from build123d import *
from OCP.BRepFilletAPI import BRepFilletAPI_MakeChamfer

# Parameters (mm, degrees)
BOSS_EXTRUDE1_DEPTH           = 6
FILLET1_R                     = 3
LPATTERN1_COUNT               = 2
LPATTERN1_PITCH               = 19
CSK_FOR_M4_SFHCS1_D           = 4.5
CSK_FOR_M4_SFHCS1_CSINK_D     = 8.96
CSK_FOR_M4_SFHCS1_CSINK_ANGLE = 90
FILLET2_R                     = 8
FILLET3_R                     = 2
CHAMFER1_SIZE                 = 3
CHAMFER1_SIZE2                = 1.732050808


# Some blends are built 0.0001 mm under size
with BuildPart() as part:
    # Sketch1 → Boss-Extrude1 (new body)
    with BuildSketch(Plane(origin=(0, 0, 0), x_dir=(1, 0, 0), z_dir=(0, 1, 0))):
        Polygon((10, 20), (16.5, 20), (16.5, 17), (10, 17), (10, 2), (16.5, 2), (16.5, -2), (10, -2), (10, -17), (16.5, -17), (16.5, -20), (10, -20), (-10, -20), (-10, 20), align=None)
    extrude(amount=BOSS_EXTRUDE1_DEPTH)

    # Fillet1
    fillet1_edges = [part.edges().sort_by_distance(p)[0] for p in [
        (16.5, 6, -18.5),
        (16.5, 0, -18.5),
        (16.5, 0, 0),
        (16.5, 0, 18.5),
        (16.5, 6, 0),
        (16.5, 6, 18.5),
    ]]
    fillet(fillet1_edges, radius=FILLET1_R - 0.0001)  # a hair under: the kernel refuses the full size

    # Sketch2 → Revolve1 (revolve)
    with BuildSketch(Plane(origin=(13.5, 0, 0), x_dir=(0, 0, -1), z_dir=(1, 0, 0))):
        with BuildLine():
            Line((-2, 3), (-2, 5.5))
            ThreePointArc((-2, 5.5), (-3.767766953, 4.767766953), (-4.5, 3))
            Line((-4.5, 3), (-2, 3))
        make_face()
    revolve1 = revolve(axis=Axis((13.5, 3, 2), (0, 0, 1)))

    # LPattern1: Revolve1 ×2
    with Locations(*[(0, 0, -i * LPATTERN1_PITCH) for i in range(1, LPATTERN1_COUNT)]):
        add(revolve1)

    # Mirror1: Revolve1 across plane
    add(revolve1.mirror(Plane.XY))

    # Mirror1 copy 1 sketch → Mirror1 copy 1 (revolve)
    with BuildSketch(Plane(origin=(13.5, 0, 19), x_dir=(0, 0, 1), z_dir=(1, 0, 0))):
        with BuildLine():
            Line((-2, -3), (-2, -5.5))
            ThreePointArc((-2, -5.5), (-3.767766953, -4.767766953), (-4.5, -3))
            Line((-4.5, -3), (-2, -3))
        make_face()
    revolve(axis=Axis((13.5, 3, 17), (0, 0, 1)))

    # CSK for M4 SFHCS1 (through all)
    with Locations(Plane(origin=(-2.75, 6, -10), x_dir=(0, 0, 1), z_dir=(0, 1, 0))):
        with Locations((0, 0), (20, 0)):
            CounterSinkHole(CSK_FOR_M4_SFHCS1_D / 2, CSK_FOR_M4_SFHCS1_CSINK_D / 2, counter_sink_angle=CSK_FOR_M4_SFHCS1_CSINK_ANGLE)

    # Fillet2
    fillet2_edges = [part.edges().sort_by_distance(p)[0] for p in [
        (-10, 3, -20),
        (-10, 3, 20),
    ]]
    fillet(fillet2_edges, radius=FILLET2_R)

    # Fillet3
    # the kernel refuses this fillet: 2 mm, written as the material it takes off along each edge
    with BuildSketch(Plane(origin=(18.5001, 6, 20), x_dir=(0, 0, -1), z_dir=(-1, 0, 0))) as fillet3_piece_1:
        with BuildLine():
            CenterArc((FILLET3_R, FILLET3_R), FILLET3_R, 180, 90)
            Line((0, FILLET3_R), (0, 0))
            Line((0, 0), (FILLET3_R, 0))
        make_face()
    extrude(amount=20.5001, mode=Mode.SUBTRACT)
    with BuildSketch(Plane(origin=(-2, 6, 12), x_dir=(-1, 0, 0), z_dir=(0, 0, -1))) as fillet3_piece_2:
        with BuildLine():
            CenterArc((8 - FILLET3_R, -FILLET3_R), FILLET3_R, 0, 90)
            Line((8, -FILLET3_R), (8, 0))
            Line((8, 0), (8 - FILLET3_R, 0))
        make_face()
    revolve(axis=Axis((-2, 6, 12), (0, 1, 0)), revolution_arc=90, mode=Mode.SUBTRACT)
    with BuildSketch(Plane(origin=(-2, 6, -12), x_dir=(0, 0, -1), z_dir=(1, 0, 0))) as fillet3_piece_3:
        with BuildLine():
            CenterArc((8 - FILLET3_R, -FILLET3_R), FILLET3_R, 0, 90)
            Line((8 - FILLET3_R, 0), (8, 0))
            Line((8, 0), (8, -FILLET3_R))
        make_face()
    revolve(axis=Axis((-2, 6, -12), (0, 1, 0)), revolution_arc=90, mode=Mode.SUBTRACT)
    with BuildSketch(Plane(origin=(-2, 6, -20), x_dir=(0, -1, 0), z_dir=(1, 0, 0))) as fillet3_piece_4:
        with BuildLine():
            CenterArc((FILLET3_R, -FILLET3_R), FILLET3_R, 90, 90)
            Line((0, -FILLET3_R), (0, 0))
            Line((0, 0), (FILLET3_R, 0))
        make_face()
    extrude(amount=20.5001, mode=Mode.SUBTRACT)
    with BuildSketch(Plane(origin=(-10, 6, 12), x_dir=(1, 0, 0), z_dir=(0, 0, -1))) as fillet3_piece_5:
        with BuildLine():
            CenterArc((FILLET3_R, FILLET3_R), FILLET3_R, 180, 90)
            Line((0, FILLET3_R), (0, 0))
            Line((0, 0), (FILLET3_R, 0))
        make_face()
    extrude(amount=24, mode=Mode.SUBTRACT)

    # Chamfer1: one chamfer whose edges measure the first distance from different faces: ONE call of the kernel's chamfer builder (chamfer() names one face for all edges)
    chamfer1_edges_1 = [part.edges().sort_by_distance(p)[0] for p in [
        (10, 6, 9.5),
    ]]
    chamfer1_side_1 = [part.faces().sort_by_distance(p)[0] for p in [
        (10, 3, 9.5),
    ]]
    chamfer1_edges_2 = [part.edges().sort_by_distance(p)[0] for p in [
        (10, 6, -9.5),
    ]]
    chamfer1_side_2 = [part.faces().sort_by_distance(p)[0] for p in [
        (10, 3, -9.5),
    ]]
    chamfer1 = BRepFilletAPI_MakeChamfer(part.part.solid().wrapped)
    for e in chamfer1_edges_1:
        chamfer1.Add(CHAMFER1_SIZE, CHAMFER1_SIZE2, e.wrapped, chamfer1_side_1[0].wrapped)  # the first distance lies on this face
    for e in chamfer1_edges_2:
        chamfer1.Add(CHAMFER1_SIZE, CHAMFER1_SIZE2, e.wrapped, chamfer1_side_2[0].wrapped)  # the first distance lies on this face
    add(Compound.cast(chamfer1.Shape()), mode=Mode.REPLACE)


solid = part.part
Verification items for the finished model (mm, model axes). A direction names the side the tool comes from. Coordinates: 2 decimals unless noted, no trailing zeros. Write each loop counter-clockwise with the first axis right and the second up, starting at its lowest first coordinate (ties: lowest second). Pieces come first, ordered by that corner, then holes. Notation, with made-up numbers: (38, 48) -> (55, 48) arc R31 cw to (55, 80) -> close; hole circle Ø9 at (-12.5, -23). An arc over 180 degrees is marked (long way). One line per item, written item: value. Start each with the question number.
Q1. Mould release check, pull along Z, two halves, no side actions. Record for faces 1 (the cylindrical face through (-7.594, 2.028, -17.719)), 2 (the cylindrical face through (-4.1, 1.9, 11.8)), 3 (the flat face through (-10, 2, 0)): pulls with the +Z half, pulls with the -Z half, needs draft (parallel to the pull), parting line crosses it, or undercut.
Q2. Cross-section at A-A on z = -10. Enter the section's corners in (x, y), and give its area (3 significant figures).
Q3. Go/stop test with flat-tipped pins: P1, Ø3.5, axis at y = 1.5, z = -10, coming from the +X side; P2, Ø3.5, axis at x = -2.75, z = -10, coming from the +Y side; P3, Ø2, axis at y = 1.5, z = 14, coming from the -X side; P4, Ø1.5, axis at x = -4.5, z = -10.5, coming from the +Y side. Record where each tip stops, or that it passes through.
Q4. Cross-section at B-B on x = 14.5. Enter the section's corners in (y, z).
Q5. Cross-section at C-C on y = 5. Enter the section's corners in (x, z).
Q6. Thickness scan on L1, parallel to X at y = 1.95, z = -10; L2, parallel to Z at x = -2.75, y = 0.95; L3, parallel to Z at x = 11.75, y = 1.5. Record the ranges inside material, lowest first. Write a range as from..to.
Q7. Access from +Z, -Z, +X, -X, +Y, -Y to the whole of each face (thin tool, end or side, straight path). Record for faces 4 (the flat face through (10, 1, -10)), 5 (the flat face through (9.122, 4.521, -9.605)), 6 (the flat face through (10.5, 3, -2)), 7 (the cylindrical face through (7.04, 5.4, -19.43)).
Checked values:
1. face 1: pulls with the -Z half
1. face 2: undercut
1. face 3: needs draft
2. outline: (-10, 0) -> (-5, 0) -> (-5, 3.77) -> (-7.23, 6) -> (-8, 6) arc R2 ccw to (-10, 4) -> close; (-0.5, 0) -> (10, 0) -> (10, 3) -> (8.27, 6) -> (1.73, 6) -> (-0.5, 3.77) -> close
2. area: 84.6 mm²
3. P1: stops at x = 10
3. P2: passes through
3. P3: stops at x = -9.94
3. P4: stops at y = 4.09
4. outline: (0.17, -20) -> (4, -20) arc R2 ccw to (5.83, -18.81) -> (5.83, -17) -> (5.29, -17) arc R2.29 ccw to (0.71, -17) -> (0.17, -17) -> close; (0.17, -2) -> (0.71, -2) arc R2.29 ccw to (5.29, -2) -> (5.83, -2) -> (5.83, 2) -> (5.29, 2) arc R2.29 ccw to (0.71, 2) -> (0.17, 2) -> close; (0.17, 17) -> (0.71, 17) arc R2.29 ccw to (5.29, 17) -> (5.83, 17) -> (5.83, 18.81) arc R2 ccw to (4, 20) -> (0.17, 20) -> close
5. outline: (-9.73, -12) arc R7.73 ccw to (-2, -19.73) -> (15.74, -19.73) -> (15.74, -17) -> (15, -17) arc R1.5 ccw to (12, -17) -> (8.85, -17) -> (8.85, -2) -> (12, -2) arc R1.5 ccw to (15, -2) -> (15.74, -2) -> (15.74, 2) -> (15, 2) arc R1.5 ccw to (12, 2) -> (8.85, 2) -> (8.85, 17) -> (12, 17) arc R1.5 ccw to (15, 17) -> (15.74, 17) -> (15.74, 19.73) -> (-2, 19.73) arc R7.73 ccw to (-9.73, 12) -> close; hole circle Ø6.96 at (-2.75, -10); hole circle Ø6.96 at (-2.75, 10)
6. L1: x = -10..-5, -0.5..10
6. L2: z = -19.96..-12.25, -7.75..7.75, 12.25..19.96
6. L3: z = -20..-16.03, -2.97..2.97, 16.03..20
7. face 4: +Y, -Y
7. face 5: +Y
7. face 6: none
7. face 7: -Z, +X, -X, +Y
